```python
from build123d import *

# Parameters (mm, degrees)
F2_SIZE  = 0.508
F3_SIZE  = 3.175
F4_R     = 32.512
F5_DEPTH = 0.508
F6_SIZE  = 0.50799
F7_SIZE  = 1


# Not quite as in the source:
# - a fillet or chamfer is up to 0.001 mm smaller than in the source, because OpenCascade refuses the exact size


with BuildPart() as f1:
    # F0 (on Right) → F1 (revolve)
    with BuildSketch(Plane.YZ):
        Polygon((0, 35.687), (0, 0), (3.175, 0), (3.175, 31.75), (22.987, 31.75), (22.987, 35.04946), (34.925, 35.04946), (34.925, 38.1), (33.69056, 38.1), (32.639, 37.04844), (21.717, 37.04844), (21.717, 35.687), align=None)
    revolve(axis=Axis((0, 1.5875, 0), (0, -1, 0)))

    # F2
    f2_edges = [f1.edges().sort_by_distance(p)[0] for p in [
        (0, 21.717, -37.04844),
        (0, 22.987, -31.75),
    ]]
    chamfer(f2_edges, length=F2_SIZE)

    # F3
    f3_edges = [f1.edges().sort_by_distance(p)[0] for p in [
        (0, 0, -35.687),
    ]]
    chamfer(f3_edges, length=F3_SIZE)

    # F4 (on face) → F5 (join)
    with BuildSketch(Plane.XZ):
        Circle(F4_R)
        with BuildLine():
            ThreePointArc((1.509855967, 6.4400210977), (1.8937491355, 6.9297046378), (2.4878198747, 7.1147556882))
            Line((2.4878198747, 7.1147556882), (5.5111409165, 7.1147556882))
            ThreePointArc((5.5111409165, 7.1147556882), (6.0757301057, 6.7551068727), (6.2165134586, 6.1006695032))
            Line((6.2165134586, 6.1006695032), (6.0470685713, 5.1900157705))
            Line((6.0470685713, 5.1900157705), (4.7878890863, 5.1900157705))
            Line((4.7878890863, 5.1900157705), (4.8664845526, 5.5916425772))
            ThreePointArc((4.8664845526, 5.5916425772), (4.836723562, 5.7383814637), (4.7118113372, 5.8209341951))
            Line((4.7118113372, 5.8209341951), (3.1333588995, 5.8209341951))
            ThreePointArc((3.1333588995, 5.8209341951), (3.0458218752, 5.7703284959), (3.0000514816, 5.6801689789))
            Line((3.0000514816, 5.6801689789), (2.9189020861, 5.2375365049))
            ThreePointArc((2.9189020861, 5.2375365049), (2.9425937197, 5.1281238685), (3.0369379092, 5.0678611733))
            Line((3.0369379092, 5.0678611733), (5.5451882072, 4.1973507032))
            ThreePointArc((5.5451882072, 4.1973507032), (5.8744055755, 3.9176753087), (5.9288027696, 3.4891390242))
            Line((5.9288027696, 3.4891390242), (5.5599426851, 1.5120476019))
            ThreePointArc((5.5599426851, 1.5120476019), (5.3557662432, 1.0797199091), (4.9655372277, 0.8034653729))
            Line((4.9655372277, 0.8034653729), (1.2082514586, 0.8034653729))
            ThreePointArc((1.2082514586, 0.8034653729), (0.6584047868, 1.1902455436), (0.4886787001, 1.8407248426))
            Line((0.4886787001, 1.8407248426), (0.7345082122, 3.0832483899))
            Line((0.7345082122, 3.0832483899), (2.1749762818, 3.0832483899))
            Line((2.1749762818, 3.0832483899), (2.0602140576, 2.5084333029))
            ThreePointArc((2.0602140576, 2.5084333029), (2.0616584556, 2.3899178369), (2.1645433735, 2.3310731631))
            Line((2.1645433735, 2.3310731631), (3.9138016291, 2.3310731631))
            ThreePointArc((3.9138016291, 2.3310731631), (4.0417506777, 2.3951715526), (4.1066328995, 2.5227249134))
            Line((4.1066328995, 2.5227249134), (4.1656503454, 2.9063397087))
            ThreePointArc((4.1656503454, 2.9063397087), (4.1228902349, 3.0507674018), (4.0033520199, 3.1424101908))
            Line((4.0033520199, 3.1424101908), (1.6647774028, 3.9686574601))
            ThreePointArc((1.6647774028, 3.9686574601), (1.2895839844, 4.3349438035), (1.2147676898, 4.8539219424))
            Line((1.2147676898, 4.8539219424), (1.509855967, 6.4400210977))
        make_face(mode=Mode.SUBTRACT)
        with BuildLine():
            Line((6.0626888962, 1.8407248426), (6.3085184083, 3.0832483899))
            Line((6.3085184083, 3.0832483899), (7.748986478, 3.0832483899))
            Line((7.748986478, 3.0832483899), (7.6342242537, 2.5084333029))
            ThreePointArc((7.6342242537, 2.5084333029), (7.6356686517, 2.3899178369), (7.7385535697, 2.3310731631))
            Line((7.7385535697, 2.3310731631), (9.4878118252, 2.3310731631))
            ThreePointArc((9.4878118252, 2.3310731631), (9.6157608738, 2.3951715526), (9.6806430956, 2.5227249134))
            Line((9.6806430956, 2.5227249134), (9.7396605415, 2.9063397087))
            ThreePointArc((9.7396605415, 2.9063397087), (9.696900431, 3.0507674018), (9.5773622161, 3.1424101908))
            Line((9.5773622161, 3.1424101908), (7.2387875989, 3.9686574601))
            ThreePointArc((7.2387875989, 3.9686574601), (6.8635941806, 4.3349438035), (6.788777886, 4.8539219424))
            Line((6.788777886, 4.8539219424), (7.0838661632, 6.4400210977))
            ThreePointArc((7.0838661632, 6.4400210977), (7.4677593317, 6.9297046378), (8.0618300708, 7.1147556882))
            Line((8.0618300708, 7.1147556882), (11.0851511126, 7.1147556882))
            ThreePointArc((11.0851511126, 7.1147556882), (11.6497403019, 6.7551068727), (11.7905236548, 6.1006695032))
            Line((11.7905236548, 6.1006695032), (11.6210787675, 5.1900157705))
            Line((11.6210787675, 5.1900157705), (10.3618992824, 5.1900157705))
            Line((10.3618992824, 5.1900157705), (10.4404947488, 5.5916425772))
            ThreePointArc((10.4404947488, 5.5916425772), (10.4107337581, 5.7383814637), (10.2858215333, 5.8209341951))
            Line((10.2858215333, 5.8209341951), (8.7073690956, 5.8209341951))
            ThreePointArc((8.7073690956, 5.8209341951), (8.6198320713, 5.7703284959), (8.5740616778, 5.6801689789))
            Line((8.5740616778, 5.6801689789), (8.4929122822, 5.2375365049))
            ThreePointArc((8.4929122822, 5.2375365049), (8.5166039159, 5.1281238685), (8.6109481053, 5.0678611733))
            Line((8.6109481053, 5.0678611733), (11.1191984033, 4.1973507032))
            ThreePointArc((11.1191984033, 4.1973507032), (11.4484157717, 3.9176753087), (11.5028129658, 3.4891390242))
            Line((11.5028129658, 3.4891390242), (11.1339528812, 1.5120476019))
            ThreePointArc((11.1339528812, 1.5120476019), (10.9297764394, 1.0797199091), (10.5395474238, 0.8034653729))
            Line((10.5395474238, 0.8034653729), (6.7822616547, 0.8034653729))
            ThreePointArc((6.7822616547, 0.8034653729), (6.232414983, 1.1902455436), (6.0626888962, 1.8407248426))
        make_face(mode=Mode.SUBTRACT)
        with BuildLine():
            Line((15.0836538523, 3.1598797068), (16.7005891971, 0.8034653729))
            Line((16.7005891971, 0.8034653729), (14.781959715, 0.8034653729))
            Line((14.781959715, 0.8034653729), (13.311708346, 3.0348771252))
            Line((13.311708346, 3.0348771252), (12.8936721012, 0.8034653729))
            Line((12.8936721012, 0.8034653729), (11.4200627431, 0.8034653729))
            Line((11.4200627431, 0.8034653729), (12.5739071518, 7.1147556882))
            Line((12.5739071518, 7.1147556882), (15.9580335021, 7.1147556882))
            ThreePointArc((15.9580335021, 7.1147556882), (16.6617692136, 6.7173463158), (16.8489553034, 5.9311278164))
            Line((16.8489553034, 5.9311278164), (16.4579637349, 3.7548521068))
            ThreePointArc((16.4579637349, 3.7548521068), (16.2392824666, 3.3522910872), (15.8235244453, 3.1598797068))
            Line((15.8235244453, 3.1598797068), (15.0836538523, 3.1598797068))
        make_face(mode=Mode.SUBTRACT)
        Polygon((26.1573679745, 7.1147556882), (28.8369659559, 7.1147556882), (26.4996811748, 0), (23.7947255373, 0), (21.1136136204, 0), (18.4020102024, 0), (20.7625944167, 7.1147556882), (23.4577525407, 7.1147556882), align=None, mode=Mode.SUBTRACT)
        with BuildLine():
            Line((15.154549852, 5.9737088159), (13.8270081952, 5.9737088159))
            Line((13.8270081952, 5.9737088159), (13.5664623231, 4.509691149))
            Line((13.5664623231, 4.509691149), (14.9684455246, 4.509691149))
            ThreePointArc((14.9684455246, 4.509691149), (15.1889852841, 4.5698286448), (15.3071191162, 4.7655291855))
            Line((15.3071191162, 4.7655291855), (15.4472859576, 5.6212851778))
            ThreePointArc((15.4472859576, 5.6212851778), (15.3812525761, 5.8642259453), (15.154549852, 5.9737088159))
        make_face()
    extrude(amount=F5_DEPTH)

    # F6 (size 0.508 in the source; OpenCascade refuses exactly that, so slightly less here)
    f6_edges = [f1.edges().sort_by_distance(p)[0] for p in [
        (0, 12.446, 35.687),
        (-32.512, -0.508, 0),
    ]]
    chamfer(f6_edges, length=F6_SIZE)

    # F7
    f7_edges = [f1.edges().sort_by_distance(p)[0] for p in [
        (0, 34.925, -35.04946),
    ]]
    chamfer(f7_edges, length=F7_SIZE)


solid = f1.part
```
Part model, mm, in its own coordinate system. A direction names the side the tool comes from. Round coordinates to 2 decimals unless told otherwise and drop trailing zeros. Loops run counter-clockwise (first coordinate to the right, second up) from the corner with the lowest first, then second, coordinate; pieces in that order, holes last. Notation, with made-up numbers: (51.25, -19.75) -> (74.25, -19.75) arc R8 ccw to (74.25, -7.75) -> close; hole circle Ø5 at (50, 73). An arc over 180 degrees is marked (long way). Use one line per item in the form item = value. Start each with the question number.
Item 1: Band-saw the part on A-A (y = 27.5). List the corners of the cut face in (x, z).
Item 2: Drop flat-ended pins along their axis: pin 1 Ø0.6 at (x, y) = (23.5, -0.5) entering from +Z; pin 2 Ø1.5 at (y, z) = (16, -10.5) entering from -X; pin 3 Ø10 at (x, y) = (18.5, 28.5) entering from +Z. Give the stop position or say it passes through.
Item 3: Drill centre lines: line 1 along Z through (x, y) = (0, 13); line 2 along Z through (x, y) = (0, 27). Where is each one in solid material? Low to high.
Item 4: Band-saw the part on B-B (y = 7.5). List the corners of the cut face in (x, z), plus the area to 3 significant figures.
Item 5: Tool access for faces 1 (the flat face through (0, -0.508, 0)), 2 (the flat face through (10, 22.987, -31)), 3 (the flat face through (9, 0, 4)): list every direction of +Z, -Z, +X, -X, +Y, -Y with a clear straight run to the whole face (end or side of a thin tool).
Data:
q1.outline = circle Ø74.1 at (0, 0); hole circle Ø70.1 at (0, 0)
q2.pin_1 = 22.28
q2.pin_2 = -34.33
q2.pin_3 = 34.5
q3.line_1 = -35.69 to -31.75, 31.75 to 35.69
q3.line_2 = -37.05 to -35.05, 35.05 to 37.05
q4.outline = circle Ø71.37 at (0, 0); hole circle Ø63.5 at (0, 0)
q4.area = 834 mm^2
q5.face_1 = +Z, -Z, +X, -X, -Y
q5.face_2 = +Y
q5.face_3 = -Y
